from build123d import *

# Parameters (mm, degrees)
EXTRUDE_1_DEPTH      = 30
SKETCH_2_R           = 1.5
CUT_EXTRUDE_1_DEPTH  = 30
EXTRUDE_2_REACH      = 36.828
EXTRUDE_2_END_RADIUS = 8
SKETCH_3_R           = 6
SKETCH_4_R           = 13
EXTRUDE_3_DEPTH      = 3
SKETCH_6_R           = 1.6
CUT_EXTRUDE_2_DEPTH  = 3


with BuildPart() as part:
    # 草图1 → 凸台-拉伸1 (new body)
    with BuildSketch(Plane.XY):
        with BuildLine():
            Line((-8, 0), (-13, 0))
            Line((-13, 0), (-13, 2))
            Line((-13, 2), (-7.745966692, 2))
            ThreePointArc((-7.745966692, 2), (0, 8), (7.745966692, 2))
            Line((7.745966692, 2), (13, 2))
            Line((13, 2), (13, 0))
            Line((13, 0), (8, 0))
            Line((8, 0), (5, 0))
            ThreePointArc((5, 0), (0, 5), (-5, 0))
            Line((-5, 0), (-8, 0))
        make_face()
    extrude(amount=EXTRUDE_1_DEPTH)

    # 草图2 → 切除-拉伸1 (cut)
    with BuildSketch(Plane(origin=(0, 2, 0), x_dir=(1, 0, 0), z_dir=(0, 1, 0))):
        with Locations(Location((10.372983346, -3.5, 0), (0, 0, 270))):
            Circle(SKETCH_2_R)
        with Locations(Location((10.372983346, -26.5, 0), (0, 0, 180))):
            Circle(SKETCH_2_R)
        with Locations(Location((-10.372983346, -26.5, 0), (0, 0, 270))):
            Circle(SKETCH_2_R)
        with Locations(Location((-10.372983346, -3.5, 0), (0, 0, 270))):
            Circle(SKETCH_2_R)
    extrude(amount=-CUT_EXTRUDE_1_DEPTH, mode=Mode.SUBTRACT)

    # 凸台-拉伸2: up to this cylinder (the profile starts outside it)
    extrude_2_end = Plane(origin=(0, 0, 15), z_dir=(0, 0, -1)) * Cylinder(EXTRUDE_2_END_RADIUS, 90.656, mode=Mode.PRIVATE)
    # 草图3 → 凸台-拉伸2 (add, up to the surface)
    with BuildSketch(Plane(origin=(0, 12, 0), x_dir=(1, 0, 0), z_dir=(0, 1, 0)), mode=Mode.PRIVATE) as extrude_2_sk1:
        with Locations(Location((0, -15, 0), (0, 0, 270))):
            Circle(SKETCH_3_R)
    extrude_2_tool1 = extrude(extrude_2_sk1.sketch, amount=-EXTRUDE_2_REACH, mode=Mode.PRIVATE) - extrude_2_end
    add(extrude_2_tool1.solids().sort_by_distance((0, 12, 15))[0])

    # 草图4 → 凸台-拉伸3 (add)
    with BuildSketch(Plane(origin=(0, 12, 0), x_dir=(1, 0, 0), z_dir=(0, 1, 0))):
        with Locations(Location((0, -15, 0), (0, 0, 270))):
            Circle(SKETCH_4_R)
    extrude(amount=EXTRUDE_3_DEPTH)

    # 草图6 → 切除-拉伸2 (cut)
    with BuildSketch(Plane(origin=(0, 15, 0), x_dir=(1, 0, 0), z_dir=(0, 1, 0))):
        with Locations(Location((10.5, -15, 0), (0, 0, 270))):
            Circle(SKETCH_6_R)
        with Locations(Location((0, -25.5, 0), (0, 0, 270))):
            Circle(SKETCH_6_R)
        with Locations(Location((-10.5, -15, 0), (0, 0, 270))):
            Circle(SKETCH_6_R)
        with Locations(Location((0, -4.5, 0), (0, 0, 270))):
            Circle(SKETCH_6_R)
    extrude(amount=-CUT_EXTRUDE_2_DEPTH, mode=Mode.SUBTRACT)


solid = part.part
The model under review builds one solid part; all positions refer to its coordinate system, in mm. A direction names the side the tool comes from. Round coordinates to 2 decimals unless told otherwise and drop trailing zeros. Loops run counter-clockwise (first coordinate to the right, second up) from the corner with the lowest first, then second, coordinate; pieces in that order, holes last. Notation, with made-up numbers: (22.25, 36.5) -> (77.25, 36.5) arc R7 cw to (77.25, 48.5) -> close; hole circle Ø10 at (46.5, 9.5). An arc over 180 degrees is marked (long way). Write item = value, one per line. Start each with the question number.
Item 1: Take a section at B-B on y = 1.25. Give the boundary of the cut face in (x, z).
Item 2: Take a section at D-D on z = 6.5. Give the boundary of the cut face in (x, y), plus the area to 3 significant figures.
Item 3: For faces 1 (the cylindrical face through (10.57, 13.52, 13.4)), 2 (the flat face through (13, 1, 15)), 3 (the cylindrical face through (-10.3, 1, 25)), 4 (the flat face through (-10, 2, 15)), 5 (the flat face through (10, 2, 15)), list the 3-axis set-ups (+Z, -Z, +X, -X, +Y, -Y) from which the entire face can be reached by the end or side of a thin tool; tool diameter is ignored.
Item 4: Mouldability with a two-part tool opening along Y and no side actions: class faces 6 (the cylindrical face through (-6.253, 4.99, 14.79)), 7 (the cylindrical face through (-2.3, 9.44, 20.54)), 8 (the flat face through (9, 0, 15)), 9 (the cylindrical face through (-0.61, 13.52, 5.98)) as released by +Y, released by -Y, zero draft, split by the parting line, or undercut.
Item 5: Take a section at A-A on z = 15. Give the boundary of the cut face in (x, y), plus the area to 3 significant figures.
Item 6: Take a section at C-C on x = -8.25. Give the boundary of the cut face in (y, z).
Item 7: To check wall thickness, follow L1, parallel to X at y = 14.1, z = 15; L2, parallel to Y at x = -6, z = 9; L3, parallel to X at y = 0.45, z = 3.5. State the ranges of each line that lie inside material, in increasing order.
Item 8: Insertion check: pin 1 (2 mm diameter, centred on x = -10, y = 13.5, fed in from +Z); pin 2 (2.5 mm diameter, centred on x = 0, z = 4.5, fed in from +Y); pin 3 (6 mm diameter, centred on y = 9.5, z = 26.5, fed in from -X). Each pin has a flat end and moves straight along its axis. Give the tip position at first contact, or say it passes through.
Result:
q1.outline = (-13, 0) -> (-4.84, 0) -> (-4.84, 30) -> (-13, 30) -> close; (4.84, 0) -> (13, 0) -> (13, 30) -> (4.84, 30) -> close; hole circle Ø3 at (-10.37, 3.5); hole circle Ø3 at (-10.37, 26.5); hole circle Ø3 at (10.37, 3.5); hole circle Ø3 at (10.37, 26.5)
q2.outline = (-13, 0) -> (-5, 0) arc R5 cw to (5, 0) -> (13, 0) -> (13, 2) -> (7.75, 2) arc R8 ccw to (-7.75, 2) -> (-13, 2) -> close; (-9.84, 12) -> (9.84, 12) -> (9.84, 15) -> (-9.84, 15) -> close
q2.area = 141 mm²
q3.face_1 = +Y
q3.face_2 = +Z, -Z, +X, +Y, -Y
q3.face_3 = +Y, -Y
q3.face_4 = +Z, -Z, -X
q3.face_5 = +Z, -Z, +X
q4.face_6 = undercut
q4.face_7 = undercut
q4.face_8 = released by -Y
q4.face_9 = zero draft
q5.outline = (-13, 0) -> (-5, 0) arc R5 cw to (5, 0) -> (13, 0) -> (13, 2) -> (7.75, 2) arc R8 ccw to (6, 5.29) -> (6, 12) -> (8.9, 12) -> (8.9, 15) -> (-8.9, 15) -> (-8.9, 12) -> (-6, 12) -> (-6, 5.29) arc R8 ccw to (-7.75, 2) -> (-13, 2) -> close; (-13, 12) -> (-12.1, 12) -> (-12.1, 15) -> (-13, 15) -> close; (12.1, 12) -> (13, 12) -> (13, 15) -> (12.1, 15) -> close
q5.area = 198 mm²
q6.outline = (0, 0) -> (2, 0) -> (2, 30) -> (0, 30) -> close; (12, 4.95) -> (15, 4.95) -> (15, 25.05) -> (12, 25.05) -> close
q7.L1 = -13 to -12.1, -8.9 to 8.9, 12.1 to 13
q7.L2 = 0 to 5.29, 12 to 15
q7.L3 = -13 to -11.87, -8.87 to -4.98, 4.98 to 8.87, 11.87 to 13
q8.pin_1 = 24.38
q8.pin_2 = 8
q8.pin_3 = -8.49
